```python
from build123d import *

# Parameters (mm, degrees)
SKETCH_6_W               = 1.25
SKETCH_6_H               = 12.35
PATTERN_CIRCULAR_1_COUNT = 4


with BuildPart() as part:
    # 草图1 → 旋转1 (revolve)
    with BuildSketch(Plane.XY, mode=Mode.PRIVATE) as revolve_1_sk:
        Polygon((6.35, 65.5), (6.35, 0), (12.35, 0), (12.35, 6), (8.975, 6), (8.975, 16), (8.475, 16.5), (8.475, 50), (8.975, 50.5), (8.975, 65.5), align=None)
    revolve(revolve_1_sk.sketch.rotate(Axis((0, 0, 0), (0, 1, 0)), 90), axis=Axis((0, 0, 0), (0, 1, 0)))

    # 草图6 → M3 螺纹孔1 (revolve, cut)
    with BuildSketch(Plane.ZX.offset(63)):
        with Locations((0.625, 6.175)):
            Rectangle(SKETCH_6_W, SKETCH_6_H)
    hole_wizard_m3_1 = revolve(axis=Axis((-6.35, 63, 0), (1, 0, 0)), mode=Mode.SUBTRACT)

    # 阵列(圆周)1: M3 螺纹孔1 ×4 about axis
    pattern_circular_1_axis = Axis((0, 65.5, 0), (0, -1, 0))
    for i in range(1, PATTERN_CIRCULAR_1_COUNT):
        add(hole_wizard_m3_1.rotate(pattern_circular_1_axis, i * 360 / PATTERN_CIRCULAR_1_COUNT), mode=Mode.SUBTRACT)


solid = part.part
```
Input: part model. Units: mm. Frame: model coordinates. A direction names the side the tool comes from. Round coordinates to 2 decimals unless told otherwise and drop trailing zeros. Order: outer loops, then holes, each group sorted by start corner. A loop starts at its lowest first (then second) coordinate and runs counter-clockwise, first axis right, second up. Notation, with made-up numbers: (49.5, 52.25) - (74.5, 52.25) arc R21 cw to (74.5, 64.25) - close; hole circle Ø3 at (40.5, -3.5). An arc over 180 degrees is marked (long way). One line per question, with ' | ' between items. Start each with the question number.
1) Cut plane D-D, the plane y = 32. Return the cut outline in (x, z) (3 decimals), then the cut area to 3 significant figures.
2) Cut plane B-B, the plane y = 63. Return the cut outline in (x, z) (3 decimals), then the cut area to 3 significant figures.
3) Ray query, probe 1 along Y at (x, z) = (7.2, 0); probe 2 along X at (y, z) = (37, 0) (3 decimals); probe 3 along X at (y, z) = (17, 3.75). Return the intervals inside material, ascending.
4) Contact query for flat-ended pins moving along their axis: P1, Ø4, axis at x = 0, y = 63, coming from the -Z side (3 decimals); P2, Ø4, axis at y = 37, z = 7, coming from the -X side; P3, Ø5, axis at x = 1.5, y = 27.5, coming from the -Z side (3 decimals). Output: stop coordinate, or through.
5) Pull-direction query (Y, two-part tool) for faces 4 (the flat face through (6, 65.5, -4)), 5 (the cylindrical face through (-0.16, 61.76, -7.62)), 6 (the cylindrical face through (7.962, 11.07, -4.141)); classes: +Y half, -Y half, draft (parallel to the pull), parting line (faces both ways), or undercut.
6) Cut plane A-A, the plane x = 0. Return the cut outline in (y, z) (3 decimals), then the cut area to 3 significant figures.
7) Cut plane C-C, the plane z = 0. Return the cut outline in (x, y) (3 decimals), then the cut area to 3 significant figures.
8) Set-up query: faces 1 (the cylindrical face through (3.86, 32.29, 5.04)), 2 (the flat face through (9.1, 6, -0.9)), 3 (the cylindrical face through (-8.403, 33.484, 1.103)). Return all of +Z, -Z, +X, -X, +Y, -Y with unobstructed straight access to the full face (end or side cutting, diameter ignored); none if empty.
Worked out:
1) outline: circle Ø16.95 at (0, 0); hole circle Ø12.7 at (0, 0) | area: 99.0 mm^2
2) outline: (-8.888, -1.25) arc R8.975 ccw to (-1.25, -8.888) - (-1.25, -6.226) arc R6.35 cw to (-6.226, -1.25) - close; (-8.888, 1.25) - (-6.226, 1.25) arc R6.35 cw to (-1.25, 6.226) - (-1.25, 8.888) arc R8.975 ccw to start; (1.25, -8.888) arc R8.975 ccw to (8.888, -1.25) - (6.226, -1.25) arc R6.35 cw to (1.25, -6.226) - close; (1.25, 6.226) arc R6.35 cw to (6.226, 1.25) - (8.888, 1.25) arc R8.975 ccw to (1.25, 8.888) - close | area: 100 mm^2
3) probe 1: y = 0 to 61.75, 64.25 to 65.5 | probe 2: x = -8.475 to -6.35, 6.35 to 8.475 | probe 3: x = -7.6 to -5.12, 5.12 to 7.6
4) P1: stops at z = -8.975 | P2: stops at x = -6.84 | P3: stops at z = -8.475
5) face 4: +Y half | face 5: undercut | face 6: draft
6) outline: (0, -12.35) - (6, -12.35) - (6, -8.975) - (16, -8.975) - (16.5, -8.475) - (50, -8.475) - (50.5, -8.975) - (61.75, -8.975) - (61.75, -6.35) - (0, -6.35) - close; (0, 6.35) - (61.75, 6.35) - (61.75, 8.975) - (50.5, 8.975) - (50, 8.475) - (16.5, 8.475) - (16, 8.975) - (6, 8.975) - (6, 12.35) - (0, 12.35) - close; (64.25, -8.975) - (65.5, -8.975) - (65.5, -6.35) - (64.25, -6.35) - close; (64.25, 6.35) - (65.5, 6.35) - (65.5, 8.975) - (64.25, 8.975) - close | area: 337 mm^2
7) outline: (-12.35, 0) - (-6.35, 0) - (-6.35, 61.75) - (-8.975, 61.75) - (-8.975, 50.5) - (-8.475, 50) - (-8.475, 16.5) - (-8.975, 16) - (-8.975, 6) - (-12.35, 6) - close; (-8.975, 64.25) - (-6.35, 64.25) - (-6.35, 65.5) - (-8.975, 65.5) - close; (6.35, 0) - (12.35, 0) - (12.35, 6) - (8.975, 6) - (8.975, 16) - (8.475, 16.5) - (8.475, 50) - (8.975, 50.5) - (8.975, 61.75) - (6.35, 61.75) - close; (6.35, 64.25) - (8.975, 64.25) - (8.975, 65.5) - (6.35, 65.5) - close | area: 337 mm^2
8) face 1: +Y, -Y | face 2: +Y | face 3: none
